from build123d import *

# Parameters (mm, degrees)
EXTRUDE_1_DEPTH     = 5
SKETCH_2_R          = 5.1
CUT_EXTRUDE_1_DEPTH = 10
SKETCH_3_R          = 14
CUT_EXTRUDE_2_DEPTH = 10
SKETCH_4_R          = 2.1
CUT_EXTRUDE_3_DEPTH = 10
CUT_EXTRUDE_4_DEPTH = 224.690634583
FILLET_1_R          = 10
SKETCH_12_R         = 1.6
CUT_EXTRUDE_5_DEPTH = 224.690634583
CUT_EXTRUDE_6_DEPTH = 10


with BuildPart() as part:
    # 草图1 → 凸台-拉伸1 (new body)
    with BuildSketch(Plane(origin=(0, 0, 0), x_dir=(1, 0, 0), z_dir=(0, 1, 0))):
        with BuildLine():
            Line((-0.25, 19.998437439), (199.71875, 22.498242119))
            ThreePointArc((199.71875, 22.498242119), (222.5, 0), (199.71875, -22.498242119))
            Line((199.71875, -22.498242119), (-0.25, -19.998437439))
            ThreePointArc((-0.25, -19.998437439), (-20, 0), (-0.25, 19.998437439))
        make_face()
    extrude(amount=EXTRUDE_1_DEPTH)

    # 草图2 → 切除-拉伸1 (cut)
    with BuildSketch(Plane(origin=(0, 5, 0), x_dir=(1, 0, 0), z_dir=(0, 1, 0))):
        with Locations(Location((0, 0, 0), (0, 0, 270))):
            Circle(SKETCH_2_R)
    extrude(amount=-CUT_EXTRUDE_1_DEPTH, mode=Mode.SUBTRACT)

    # 草图3 → 切除-拉伸2 (cut)
    with BuildSketch(Plane(origin=(0, 5, 0), x_dir=(1, 0, 0), z_dir=(0, 1, 0))):
        with Locations(Location((200, 0, 0), (0, 0, 270))):
            Circle(SKETCH_3_R)
    extrude(amount=-CUT_EXTRUDE_2_DEPTH, mode=Mode.SUBTRACT)

    # 草图4 → 切除-拉伸3 (cut)
    with BuildSketch(Plane(origin=(0, 5, 0), x_dir=(1, 0, 0), z_dir=(0, 1, 0))):
        with Locations(Location((0, 12, 0), (0, 0, 270))):
            Circle(SKETCH_4_R)
        with Locations(Location((10.392304845, 6, 0), (0, 0, 270))):
            Circle(SKETCH_4_R)
        with Locations(Location((10.392304845, -6, 0), (0, 0, 270))):
            Circle(SKETCH_4_R)
        with Locations(Location((0, -12, 0), (0, 0, 270))):
            Circle(SKETCH_4_R)
        with Locations(Location((-10.392304845, -6, 0), (0, 0, 270))):
            Circle(SKETCH_4_R)
        with Locations(Location((-10.392304845, 6, 0), (0, 0, 270))):
            Circle(SKETCH_4_R)
    extrude(amount=-CUT_EXTRUDE_3_DEPTH, mode=Mode.SUBTRACT)

    # 草图10 → 切除-拉伸4 (cut, through all)
    with BuildSketch(Plane(origin=(0, 5, 0), x_dir=(1, 0, 0), z_dir=(0, 1, 0))):
        with BuildLine():
            Line((19.75, 15), (169.71875, 15))
            ThreePointArc((169.71875, 15), (184.427162899, 19.915742901), (199.71875, 22.498242119))
            Line((199.71875, 22.498242119), (-0.25, 19.998437439))
            ThreePointArc((-0.25, 19.998437439), (9.879148371, 18.015973695), (19.75, 15))
        make_face()
        with BuildLine():
            Line((19.75, -15), (169.71875, -15))
            ThreePointArc((169.71875, -15), (184.427162899, -19.915742901), (199.71875, -22.498242119))
            Line((199.71875, -22.498242119), (-0.25, -19.998437439))
            ThreePointArc((-0.25, -19.998437439), (9.879148371, -18.015973695), (19.75, -15))
        make_face()
    extrude(amount=-CUT_EXTRUDE_4_DEPTH, mode=Mode.SUBTRACT)

    # 圆角1
    fillet_1_edges = [part.edges().sort_by_distance(p)[0] for p in [
        (169.71875, 2.5, 15),
        (19.75, 2.5, 15),
        (19.75, 2.5, -15),
        (169.71875, 2.5, -15),
    ]]
    fillet(fillet_1_edges, radius=FILLET_1_R)

    # 草图12 → 切除-拉伸5 (cut, through all)
    with BuildSketch(Plane(origin=(0, 5, 0), x_dir=(1, 0, 0), z_dir=(0, 1, 0))):
        with Locations(Location((160, 0, 0), (0, 0, 270))):
            Circle(SKETCH_12_R)
        with Locations(Location((60, 0, 0), (0, 0, 270))):
            Circle(SKETCH_12_R)
        with Locations(Location((175, 0, 0), (0, 0, 270))):
            Circle(SKETCH_12_R)
        with BuildLine():
            Line((76.690146779, 10), (143.309853221, 10))
            ThreePointArc((143.309853221, 10), (144.993003562, 8.426306348), (143.535868598, 6.64129529))
            Line((143.535868598, 6.64129529), (112.102965186, 2.39880546))
            ThreePointArc((112.102965186, 2.39880546), (109.999758761, 2.251989281), (107.896074318, 2.391789195))
            Line((107.896074318, 2.391789195), (76.464131402, 6.64129529))
            ThreePointArc((76.464131402, 6.64129529), (75.006996438, 8.426306348), (76.690146779, 10))
        make_face()
        with BuildLine():
            Line((65, 3.615503909), (65, -3.615503909))
            ThreePointArc((65, -3.615503909), (65.713191903, -5.175920839), (67.359810975, -5.657781105))
            Line((67.359810975, -5.657781105), (100.428751598, -0.862135837))
            ThreePointArc((100.428751598, -0.862135837), (101.174879309, 0), (100.428751598, 0.862135837))
            Line((100.428751598, 0.862135837), (67.359810975, 5.657781105))
            ThreePointArc((67.359810975, 5.657781105), (65.713191903, 5.175920839), (65, 3.615503909))
        make_face()
        with BuildLine():
            Line((155, 3.615503909), (155, -3.615503909))
            ThreePointArc((155, -3.615503909), (154.286808097, -5.175920839), (152.640189025, -5.657781105))
            Line((152.640189025, -5.657781105), (119.571248402, -0.862135837))
            ThreePointArc((119.571248402, -0.862135837), (118.825120691, 0), (119.571248402, 0.862135837))
            Line((119.571248402, 0.862135837), (152.640189025, 5.657781105))
            ThreePointArc((152.640189025, 5.657781105), (154.286808097, 5.175920839), (155, 3.615503909))
        make_face()
        with BuildLine():
            Line((76.464131402, -6.64129529), (107.896074318, -2.391789195))
            ThreePointArc((107.896074318, -2.391789195), (109.999758761, -2.251989281), (112.102965186, -2.39880546))
            Line((112.102965186, -2.39880546), (143.535868598, -6.64129529))
            ThreePointArc((143.535868598, -6.64129529), (144.993003562, -8.426306348), (143.309853221, -10))
            Line((143.309853221, -10), (76.690146779, -10))
            ThreePointArc((76.690146779, -10), (75.006996438, -8.426306348), (76.464131402, -6.64129529))
        make_face()
    extrude(amount=-CUT_EXTRUDE_5_DEPTH, mode=Mode.SUBTRACT)

    # 草图13 → 切除-拉伸6 (cut)
    with BuildSketch(Plane(origin=(0, 5, 0), x_dir=(1, 0, 0), z_dir=(0, 1, 0))):
        with BuildLine():
            Line((20.970819312, 8.785118289), (49.029180688, 8.785118289))
            ThreePointArc((49.029180688, 8.785118289), (50.351263939, 7.681791354), (49.502305324, 6.183624568))
            Line((49.502305324, 6.183624568), (39.957431091, 2.113629648))
            ThreePointArc((39.957431091, 2.113629648), (35.035801099, 1.547966117), (30.182224549, 2.540544414))
            Line((30.182224549, 2.540544414), (20.497694676, 6.183624568))
            ThreePointArc((20.497694676, 6.183624568), (19.648736061, 7.681791354), (20.970819312, 8.785118289))
        make_face()
        with BuildLine():
            Line((16.490400657, 4.317991857), (16.490400657, -4.317991857))
            ThreePointArc((16.490400657, -4.317991857), (17.156548552, -5.478408553), (18.494540137, -5.488330518))
            Line((18.494540137, -5.488330518), (25.642155827, -1.455347803))
            ThreePointArc((25.642155827, -1.455347803), (26.492021725, 0), (25.642155827, 1.455347803))
            Line((25.642155827, 1.455347803), (18.494540137, 5.488330518))
            ThreePointArc((18.494540137, 5.488330518), (17.156548552, 5.478408553), (16.490400657, 4.317991857))
        make_face()
        with BuildLine():
            Line((53.509599343, 4.317991857), (53.509599343, -4.317991857))
            ThreePointArc((53.509599343, -4.317991857), (52.843451448, -5.478408553), (51.505459863, -5.488330518))
            Line((51.505459863, -5.488330518), (44.357844173, -1.455347803))
            ThreePointArc((44.357844173, -1.455347803), (43.507978275, 0), (44.357844173, 1.455347803))
            Line((44.357844173, 1.455347803), (51.505459863, 5.488330518))
            ThreePointArc((51.505459863, 5.488330518), (52.843451448, 5.478408553), (53.509599343, 4.317991857))
        make_face()
        with BuildLine():
            Line((20.497694676, -6.183624568), (30.182224549, -2.540544414))
            ThreePointArc((30.182224549, -2.540544414), (35.035801099, -1.547966117), (39.957431091, -2.113629648))
            Line((39.957431091, -2.113629648), (49.502305324, -6.183624568))
            ThreePointArc((49.502305324, -6.183624568), (50.351263939, -7.681791354), (49.029180688, -8.785118289))
            Line((49.029180688, -8.785118289), (20.970819312, -8.785118289))
            ThreePointArc((20.970819312, -8.785118289), (19.648736061, -7.681791354), (20.497694676, -6.183624568))
        make_face()
    extrude(amount=-CUT_EXTRUDE_6_DEPTH, mode=Mode.SUBTRACT)


solid = part.part
Geometry check sheet. Reference: the model listing, model coordinates, mm. A direction names the side the tool comes from. Round coordinates to 2 decimals unless told otherwise and drop trailing zeros. Write each loop counter-clockwise with the first axis right and the second up, starting at its lowest first coordinate (ties: lowest second). Pieces come first, ordered by that corner, then holes. Notation, with made-up numbers: (-22.75, 4.25) -> (-7.75, 4.25) arc R14 cw to (-7.75, 22.25) -> close; hole circle Ø6 at (18, 70.25). An arc over 180 degrees is marked (long way). One line per item, written item: value. Start each with the question number.
(1) Draft check along Z on faces 1 (the cylindrical face through (185.14, 2.54, -20.09)), 2 (the cylindrical face through (8.96, 2.54, 18.24)), 3 (the flat face through (110, 3, 10)). Enter one of: +Z half, -Z half, draft (parallel to the pull), parting line (faces both ways), or undercut.
(2) Go/stop test with flat-tipped pins: pin 1 Ø2 at (x, y) = (127.5, 4) entering from +Z; pin 2 Ø2 at (x, y) = (190, 3.5) entering from +Z; pin 3 Ø1.5 at (y, z) = (2, -1) entering from -X. Record where each tip stops, or that it passes through.
(3) Cross-section at C-C, the plane y = 3.75. Give the number of separate pieces and of enclosed holes in the cut face, and give its area (3 significant figures).
(4) Access from +Z, -Z, +X, -X, +Y, -Y to the whole of each face (thin tool, end or side, straight path). Record for faces 4 (the cylindrical face through (169.61, 2.465, -15.176)), 5 (the flat face through (94, 3, 15)), 6 (the flat face through (91.96, 2.535, 4.546)).
(5) Cross-section at B-B, the plane x = 95. Record the cut outline in (y, z), and give its area (3 significant figures).
(6) Cross-section at A-A, the plane z = 12. Record the cut outline in (x, y).
(7) Scan lines: line 1 (X direction, y = 1.7, z = -12); line 2 (Z direction, x = 30, y = 2.6); line 3 (Z direction, x = 120.5, y = 3.05). Record each from-to range of solid material in increasing order. Write a range as [from, to].
Answer:
1. face 1: -Z half
1. face 2: +Z half
1. face 3: undercut
2. pin 1: z = 15
2. pin 2: z = 21.33
2. pin 3: x = -20
3. separate pieces: 1
3. enclosed holes: 19
3. area: 5,300 mm²
4. face 4: -Z, +Y, -Y
4. face 5: +Z, +Y, -Y
4. face 6: +Y, -Y
5. outline: (0, -15) -> (5, -15) -> (5, -10) -> (0, -10) -> close; (0, -4.14) -> (5, -4.14) -> (5, -1.65) -> (0, -1.65) -> close; (0, 1.65) -> (5, 1.65) -> (5, 4.14) -> (0, 4.14) -> close; (0, 10) -> (5, 10) -> (5, 15) -> (0, 15) -> close
5. area: 74.9 mm²
6. outline: (-16, 0) -> (-2.1, 0) -> (-2.1, 5) -> (-16, 5) -> close; (2.1, 0) -> (192.79, 0) -> (192.79, 5) -> (2.1, 5) -> close; (207.21, 0) -> (219.03, 0) -> (219.03, 5) -> (207.21, 5) -> close
7. line 1: [-16, -2.1], [2.1, 192.79], [207.21, 219.03]
7. line 2: [-15, -8.79], [-2.61, 2.61], [8.79, 15]
7. line 3: [-15, -10], [-3.53, -1], [1, 3.53], [10, 15]
